```python
from build123d import *

# Parameters (mm, degrees)
F0_W     = 12
F0_H     = 15
F1_DEPTH = 2.35
F2_W     = 1.5
F2_H     = 1.6
F3_DEPTH = 1.7
F4_W     = 0.6
F4_H     = 0.4
F5_DEPTH = 2.5


with BuildPart() as f1:
    # F0 (on Front) → F1 (new body, symmetric)
    with BuildSketch(Plane.XZ):
        Rectangle(F0_W, F0_H)
    extrude(amount=F1_DEPTH, both=True)

    # F2 (on face) → F3 (cut)
    with BuildSketch(Plane.XZ.offset(2.35)):
        with BuildLine():
            Line((-6, 6.4), (-6, 5))
            ThreePointArc((-6, 5), (-5.3, 5.7), (-6, 6.4))
        make_face()
        with Locations((-3.45, 2.4)):
            Rectangle(F2_W, F2_H)
        with Locations((-1.15, 2.4)):
            Rectangle(F2_W, F2_H)
        with Locations((1.15, 2.4)):
            Rectangle(F2_W, F2_H)
        with Locations((3.45, 2.4)):
            Rectangle(F2_W, F2_H)
        with Locations((3.45, 0)):
            Rectangle(F2_W, F2_H)
        with Locations((1.15, 0)):
            Rectangle(F2_W, F2_H)
        with Locations((-1.15, 0)):
            Rectangle(F2_W, F2_H)
        with Locations((-3.45, 0)):
            Rectangle(F2_W, F2_H)
        with Locations((-3.45, -2.4)):
            Rectangle(F2_W, F2_H)
        with Locations((-1.15, -2.4)):
            Rectangle(F2_W, F2_H)
        with Locations((1.15, -2.4)):
            Rectangle(F2_W, F2_H)
        with Locations((3.45, -2.4)):
            Rectangle(F2_W, F2_H)
        with BuildLine():
            Line((6, -6.4), (6, -5))
            ThreePointArc((6, -5), (5.3, -5.7), (6, -6.4))
        make_face()
        with BuildLine():
            Line((-6, -5), (-6, -6.4))
            ThreePointArc((-6, -6.4), (-5.3, -5.7), (-6, -5))
        make_face()
        with BuildLine():
            ThreePointArc((6, 6.4), (5.3, 5.7), (6, 5))
            Line((6, 5), (6, 6.4))
        make_face()
        with BuildLine():
            ThreePointArc((-0.7, 7.5), (0, 6.8), (0.7, 7.5))
            Line((0.7, 7.5), (-0.7, 7.5))
        make_face()
    extrude(amount=-F3_DEPTH, mode=Mode.SUBTRACT)

    # F4 (on face) → F5 (join)
    with BuildSketch(Plane(origin=(0, 0, -7.5), x_dir=(1, 0, 0), z_dir=(0, 0, -1))):
        with Locations((-3.81, -1.15)):
            Rectangle(F4_W, F4_H)
        with Locations((-1.27, -1.15)):
            Rectangle(F4_W, F4_H)
        with Locations((1.27, -1.15)):
            Rectangle(F4_W, F4_H)
        with Locations((3.81, -1.15)):
            Rectangle(F4_W, F4_H)
    extrude(amount=F5_DEPTH)


solid = f1.part
```
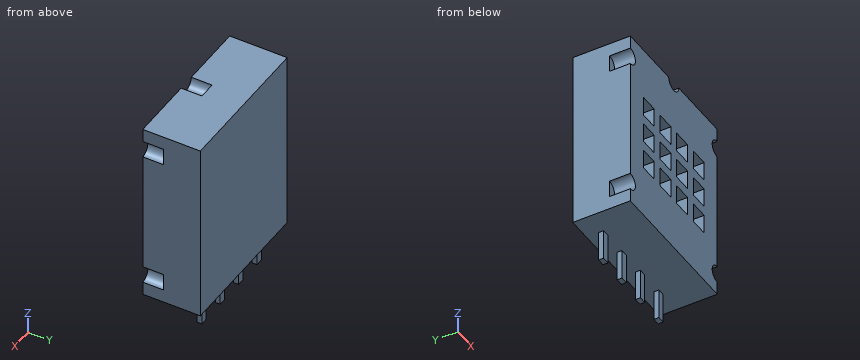
Read the model definition and answer for the solid it produces. Units are mm, in the model's axes. Give positions to 0.01 mm unless a question says otherwise; leave off trailing zeros. Write each loop counter-clockwise with the first axis right and the second up, starting at its lowest first coordinate (ties: lowest second). Pieces come first, ordered by that corner, then holes. Notation, with made-up numbers: (88, 7) - (124, 7) arc R25 ccw to (124, 41) - close; hole circle Ø8 at (-31, -5). An arc over 180 degrees is marked (long way). Write item = value, one per line. Start each with the question number.
Item 1: Find section D-D (y = 1.55). Give the vertices of the cut face in (x, z), then the cut area to 3 significant figures.
Item 2: Find section B-B (x = -3.75). Give the vertices of the cut face in (y, z), then the cut area to 3 significant figures.
Item 3: Find the intervals of material crossed by probe 1 along X at (y, z) = (-1, -2.75); probe 2 along Z at (x, y) = (3.25, -0.8); probe 3 along Z at (x, y) = (-5.5, -1.9), in increasing order. Write a range as [from, to].
Item 4: Find section C-C (y = -1.2). State how many separate pieces and enclosed holes the cut face has, then the cut area to 3 significant figures.
Item 5: Find section A-A (z = -2.25). Give the vertices of the cut face in (x, y).
Item 6: This flat-tipped pin is pushed along its axis until it touches: P1, Ø0.8, axis at x = 3.5, y = -2, coming from the -Z side. Where does it stop, or does it pass through?
Response:
q1.outline = (-6, -7.5) - (6, -7.5) - (6, 7.5) - (-6, 7.5) - close
q1.area = 180 mm²
q2.outline = (-2.35, -7.5) - (0.95, -7.5) - (0.95, -10) - (1.35, -10) - (1.35, -7.5) - (2.35, -7.5) - (2.35, 7.5) - (-2.35, 7.5) - (-2.35, 3.2) - (-0.65, 3.2) - (-0.65, 1.6) - (-2.35, 1.6) - (-2.35, 0.8) - (-0.65, 0.8) - (-0.65, -0.8) - (-2.35, -0.8) - (-2.35, -1.6) - (-0.65, -1.6) - (-0.65, -3.2) - (-2.35, -3.2) - close
q2.area = 63.3 mm²
q3.probe_1 = [-6, -4.2], [-2.7, -1.9], [-0.4, 0.4], [1.9, 2.7], [4.2, 6]
q3.probe_2 = [-7.5, -3.2], [-1.6, -0.8], [0.8, 1.6], [3.2, 7.5]
q3.probe_3 = [-7.5, -6.19], [-5.21, 5.21], [6.19, 7.5]
q4.separate_pieces = 1
q4.enclosed_holes = 12
q4.area = 147 mm²
q5.outline = (-6, -2.35) - (-4.2, -2.35) - (-4.2, -0.65) - (-2.7, -0.65) - (-2.7, -2.35) - (-1.9, -2.35) - (-1.9, -0.65) - (-0.4, -0.65) - (-0.4, -2.35) - (0.4, -2.35) - (0.4, -0.65) - (1.9, -0.65) - (1.9, -2.35) - (2.7, -2.35) - (2.7, -0.65) - (4.2, -0.65) - (4.2, -2.35) - (6, -2.35) - (6, 2.35) - (-6, 2.35) - close
q6.P1 = -7.5
